```python
from build123d import *

# Parameters (mm, degrees)
BOSS_EXTRUDE1_OUTLINE_R   = 36
BOSS_EXTRUDE1_OUTLINE_R_2 = 9.5
BOSS_EXTRUDE1_OUTLINE_W   = 16
BOSS_EXTRUDE1_OUTLINE_H   = 68.6
BOSS_EXTRUDE1_DEPTH       = 20
SKETCH4_R                 = 3.999999999999999
CUT_EXTRUDE6_DEPTH        = 55.699177324709375
SKETCH5_R                 = 1.5000000000000009
CUT_EXTRUDE2_DEPTH        = 20
CUT_EXTRUDE4_DEPTH        = 55.699177324709375
CUT_EXTRUDE4_DEPTH_BACK   = 55.699177324709375
SKETCH6_R                 = 3.0999999999999988
CUT_EXTRUDE5_DEPTH        = 55.699177324709375
CUT_EXTRUDE5_DEPTH_BACK   = 55.699177324709375
BOSS_EXTRUDE2_OUTLINE_R   = 1.5
BOSS_EXTRUDE2_OUTLINE_R_2 = 3.1
BOSS_EXTRUDE2_OUTLINE_W   = 16
BOSS_EXTRUDE2_OUTLINE_H   = 68.6
BOSS_EXTRUDE2_OUTLINE_R_3 = 4
BOSS_EXTRUDE2_DEPTH       = 3
SKETCH9_3_W               = 16
SKETCH9_3_H               = 68.6
SKETCH9_3_W_2             = 15
SKETCH9_3_H_2             = 30
BOSS_EXTRUDE3_DEPTH       = 3
CIRPATTERN1_DEPTH         = 23
FILLET1_R                 = 5
FILLET2_R                 = 3


# Read off the part's stored shape, not the designer's step: Boss-Extrude1, Boss-Extrude2, CirPattern1
with BuildPart() as part:
    # Boss-Extrude1 outline → Boss-Extrude1 (new body)
    with BuildSketch(Plane(origin=(0, 0, 0), x_dir=(1, 0, 0), z_dir=(0, 1, 0))):
        Circle(BOSS_EXTRUDE1_OUTLINE_R)
        with Locations((-24.625, 0)):
            Circle(BOSS_EXTRUDE1_OUTLINE_R_2, mode=Mode.SUBTRACT)
        Rectangle(BOSS_EXTRUDE1_OUTLINE_W, BOSS_EXTRUDE1_OUTLINE_H, mode=Mode.SUBTRACT)
        with Locations((24.625, 0)):
            Circle(BOSS_EXTRUDE1_OUTLINE_R_2, mode=Mode.SUBTRACT)
    extrude(amount=BOSS_EXTRUDE1_DEPTH)

    # Sketch4 → Cut-Extrude6 (cut, through all)
    with BuildSketch(Plane(origin=(0, 20, 0), x_dir=(1, 0, 0), z_dir=(0, 1, 0))):
        with Locations((-24.625, 9.500000000000002)):
            Circle(SKETCH4_R)
        with Locations((24.625, -9.500000000000002)):
            Circle(SKETCH4_R)
    extrude(amount=-CUT_EXTRUDE6_DEPTH, mode=Mode.SUBTRACT)

    # Sketch5 → Cut-Extrude2 (cut)
    with BuildSketch(Plane(origin=(0, 20, 0), x_dir=(1, 0, 0), z_dir=(0, 1, 0))):
        with Locations(Location((-21.667008816788154, 18.18077910688168, 0), (0, 0, 270))):
            Circle(SKETCH5_R)
        with Locations(Location((18.180779106881676, 21.667008816788137, 0), (0, 0, 270))):
            Circle(SKETCH5_R)
        with Locations(Location((-18.18077910688169, -21.66700881678815, 0), (0, 0, 270))):
            Circle(SKETCH5_R)
        with Locations(Location((21.667008816788147, -18.180779106881687, 0), (0, 0, 270))):
            Circle(SKETCH5_R)
    extrude(amount=-CUT_EXTRUDE2_DEPTH, mode=Mode.SUBTRACT)

    # Sketch6 → Cut-Extrude4 (cut, two sides: drawn at the far end of the back side and taken through both)
    with BuildSketch(Plane(origin=(0, 20, 0), x_dir=(1, 0, 0), z_dir=(0, 1, 0)).offset(-CUT_EXTRUDE4_DEPTH_BACK)):
        with Locations(Location((-24.68172400785648, -14.250000000000037, 0), (0, 0, 270))):
            Circle(SKETCH6_R)
        with Locations(Location((24.68172400785648, 14.25000000000004, 0), (0, 0, 270))):
            Circle(SKETCH6_R)
    extrude(amount=CUT_EXTRUDE4_DEPTH + CUT_EXTRUDE4_DEPTH_BACK, mode=Mode.SUBTRACT)

    # Sketch7 → Cut-Extrude5 (cut, two sides: drawn at the far end of the back side and taken through both)
    with BuildSketch(Plane(origin=(0, 20, 0), x_dir=(1, 0, 0), z_dir=(0, 1, 0)).offset(-CUT_EXTRUDE5_DEPTH_BACK)):
        with BuildLine():
            ThreePointArc((-25.25978035738815, 25.650409281266985), (-17.20729309053125, 24.574561328669844), (-15.46414662353581, 32.50938586325165))
            ThreePointArc((-15.46414662353581, 32.50938586325165), (-20.64875170863751, 29.48947359440382), (-25.25978035738815, 25.650409281266985))
        make_face()
    extrude(amount=CUT_EXTRUDE5_DEPTH + CUT_EXTRUDE5_DEPTH_BACK, mode=Mode.SUBTRACT)

    # Boss-Extrude2 outline → Boss-Extrude2 (add)
    with BuildSketch(Plane(origin=(0, 20, 0), x_dir=(1, 0, 0), z_dir=(0, 1, 0))):
        with BuildLine():
            ThreePointArc((-25.259780357, 25.650409281), (20.648751711, -29.489473593), (-15.464146624, 32.509385863))
            ThreePointArc((-15.464146624, 32.509385863), (-17.207293091, 24.574561329), (-25.259780357, 25.650409281))
        make_face()
        with Locations((-18.180779107, -21.667008817)):
            Circle(BOSS_EXTRUDE2_OUTLINE_R, mode=Mode.SUBTRACT)
        with Locations((-24.681724008, -14.25)):
            Circle(BOSS_EXTRUDE2_OUTLINE_R_2, mode=Mode.SUBTRACT)
        Rectangle(BOSS_EXTRUDE2_OUTLINE_W, BOSS_EXTRUDE2_OUTLINE_H, mode=Mode.SUBTRACT)
        with Locations((21.667008817, -18.180779107)):
            Circle(BOSS_EXTRUDE2_OUTLINE_R, mode=Mode.SUBTRACT)
        with Locations((24.625, -9.5)):
            Circle(BOSS_EXTRUDE2_OUTLINE_R_3, mode=Mode.SUBTRACT)
        with Locations((-24.625, 9.5)):
            Circle(BOSS_EXTRUDE2_OUTLINE_R_3, mode=Mode.SUBTRACT)
        with Locations((-21.667008817, 18.180779107)):
            Circle(BOSS_EXTRUDE2_OUTLINE_R, mode=Mode.SUBTRACT)
        with Locations((24.681724008, 14.25)):
            Circle(BOSS_EXTRUDE2_OUTLINE_R_2, mode=Mode.SUBTRACT)
        with Locations((18.180779107, 21.667008817)):
            Circle(BOSS_EXTRUDE2_OUTLINE_R, mode=Mode.SUBTRACT)
    extrude(amount=BOSS_EXTRUDE2_DEPTH)

    # Sketch9<3> → Boss-Extrude3 (add)
    with BuildSketch(Plane(origin=(0, 20, 0), x_dir=(1, 0, 0), z_dir=(0, 1, 0))):
        Rectangle(SKETCH9_3_W, SKETCH9_3_H)
        Rectangle(SKETCH9_3_W_2, SKETCH9_3_H_2, mode=Mode.SUBTRACT)
    extrude(amount=BOSS_EXTRUDE3_DEPTH)

    # CirPattern1 outline → CirPattern1 (cut)
    with BuildSketch(Plane(origin=(0, 0, 0), x_dir=(1, 0, 0), z_dir=(0, 1, 0))):
        with BuildLine():
            ThreePointArc((15.464146624, -32.509385863), (20.648751709, -29.489473594), (25.259780357, -25.650409281))
            ThreePointArc((25.259780357, -25.650409281), (17.207293091, -24.574561329), (15.464146624, -32.509385863))
        make_face()
    extrude(amount=CIRPATTERN1_DEPTH, mode=Mode.SUBTRACT)

    # Fillet1
    fillet1_edges = [part.edges().sort_by_distance(p)[0] for p in [
        (7.499999999999997, 21.5, -14.999999999999998),
        (7.499999999999997, 21.5, 15.000000000000002),
        (-7.500000000000003, 21.5, 15.000000000000002),
        (-7.500000000000003, 21.5, -14.999999999999998),
    ]]
    fillet(fillet1_edges, radius=FILLET1_R)

    # Fillet2
    fillet2_edges = [part.edges().sort_by_distance(p)[0] for p in [
        (25.259780357000004, 10, 25.650409281),
        (15.464146623999998, 10, 32.509385863),
        (-25.259780357388152, 10, -25.650409281266985),
        (-15.46414662353581, 10, -32.50938586325165),
    ]]
    fillet(fillet2_edges, radius=FILLET2_R)


solid = part.part
```
Verification items for the finished model (mm, model axes). A direction names the side the tool comes from. Coordinates: 2 decimals unless noted, no trailing zeros. Write each loop counter-clockwise with the first axis right and the second up, starting at its lowest first coordinate (ties: lowest second). Pieces come first, ordered by that corner, then holes. Notation, with made-up numbers: M 3.25,61.5 L 60.25,61.5 A14 ccw 60.25,83.5 Z; hole C -36,89 d9. An arc over 180 degrees is marked long. One line per item, written item: value.
Item 1: Section check C-C, the plane y = 16. State how many separate pieces and enclosed holes the cut face has, plus the area to 3 significant figures.
Check sheet entries:
separate pieces: 1
enclosed holes: 9
area: 2,150 mm^2
Item 2: Section check B-B, the plane x = -6. Record the boundary of the cut face in (y, z), plus the area to 3 significant figures.
Check sheet entries:
outline: M 0,-35.5 L 23,-35.5 L 23,-13.57 L 20,-13.57 L 20,-34.3 L 0,-34.3 Z; M 0,34.3 L 20,34.3 L 20,13.57 L 23,13.57 L 23,35.5 L 0,35.5 Z
area: 179 mm^2
Item 3: Gauge pin test, flat ends, axial feed: pin 1 Ø5 at (y, z) = (19, -3.5) entering from -X; pin 2 Ø1.5 at (x, z) = (-22.5, -10) entering from -Y; pin 3 Ø6 at (y, z) = (11, 5.5) entering from +X; pin 4 Ø3 at (y, z) = (19, -22.5) entering from +X. Record the tip position at first contact, or that the pin passes through.
Check sheet entries:
pin 1: stops at x = -35.99
pin 2: passes through
pin 3: stops at x = 35.91
pin 4: stops at x = 29.24
Item 4: Scan lines: line 1 along X through (y, z) = (5, 0) (3 decimals); line 2 along X through (y, z) = (14.5, -6); line 3 along Z through (x, y) = (-26.5, 9.75). Record each from-to range of solid material in increasing order.
Check sheet entries:
line 1: x = -36 to -34.125, -15.125 to -8, 8 to 15.125, 34.125 to 36
line 2: x = -35.5 to -31.99, -17.26 to -8, 8 to 17.26, 31.99 to 35.5
line 3: z = -24.16 to -13.03, 9.31 to 11.74, 16.76 to 24.37
Item 5: Access from +Z, -Z, +X, -X, +Y, -Y to the whole of each face (thin tool, end or side, straight path). Record for faces 3 (the flat face through (-25, 20, 0)), 4 (the flat face through (0, 21, -15)).
Check sheet entries:
face 3: -Y
face 4: +Y, -Y
Item 6: Mould release check, pull along X, two halves, no side actions. Record for faces 1 (the flat face through (0, 10, 34.3)), 2 (the flat face through (-9, 23, -1)): pulls with the +X half, pulls with the -X half, needs draft (parallel to the pull), parting line crosses it, or undercut.
Check sheet entries:
face 1: undercut
face 2: needs draft
Item 7: Section check A-A, the plane z = 0. Record the boundary of the cut face in (x, y) (3 decimals).
Check sheet entries:
outline: M -36,0 L -34.125,0 L -34.125,20 L -15.125,20 L -15.125,0 L -8,0 L -8,20 L -7.5,20 L -7.5,23 L -36,23 Z; M 7.5,20 L 8,20 L 8,0 L 15.125,0 L 15.125,20 L 34.125,20 L 34.125,0 L 36,0 L 36,23 L 7.5,23 Z
